```python
from build123d import *

# Parameters (mm, degrees)
BOSS_EXTRUDE1_DEPTH = 53.1
SKETCH3_W           = 0.955506131
SKETCH3_H           = 0.5
BOSS_EXTRUDE3_DEPTH = 5
BOSS_EXTRUDE4_DEPTH = 6
BOSS_EXTRUDE5_DEPTH = 5.84


with BuildPart() as part:
    # Sketch1 → Boss-Extrude1 (new body)
    with BuildSketch(Plane(origin=(0, 0, 0), x_dir=(0, 0, -1), z_dir=(1, 0, 0))):
        Polygon((0, 0), (12.5, 0), (12.5, 3.577441077), (3.577441077, 3.577441077), (3.577441077, 12.5), (0, 12.5), align=None)
    extrude(amount=BOSS_EXTRUDE1_DEPTH)

    # Sketch3 → Boss-Extrude3 (add)
    with BuildSketch(Plane.XZ):
        with Locations((1.917753066, -9.5)):
            Rectangle(SKETCH3_W, SKETCH3_H)
        with Locations((4.142246935, -9.5)):
            Rectangle(SKETCH3_W, SKETCH3_H)
        with Locations((48.957753066, -9.5)):
            Rectangle(SKETCH3_W, SKETCH3_H)
        with Locations((51.182246935, -9.5)):
            Rectangle(SKETCH3_W, SKETCH3_H)
    extrude(amount=BOSS_EXTRUDE3_DEPTH)

    # Sketch4 → Boss-Extrude4 (add)
    with BuildSketch(Plane.XY):
        Polygon((4.177995884, 4.261612802), (5.325991768, 6.25), (4.177995884, 8.238387198), (1.882004116, 8.238387198), (0.734008232, 6.25), (1.882004116, 4.261612802), align=None)
        Polygon((51.217995884, 4.261612802), (52.365991768, 6.25), (51.217995884, 8.238387198), (48.922004116, 8.238387198), (47.774008232, 6.25), (48.922004116, 4.261612802), align=None)
    extrude(amount=BOSS_EXTRUDE4_DEPTH)

    # Sketch6 → Boss-Extrude5 (add)
    with BuildSketch(Plane.XY):
        with BuildLine():
            Line((9.7116, 10.93), (43.3884, 10.93))
            ThreePointArc((43.3884, 10.93), (45.795005223, 9.807781555), (46.482272037, 7.242866885))
            Line((46.482272037, 7.242866885), (45.939749183, 4.166066885))
            ThreePointArc((45.939749183, 4.166066885), (44.8652587, 2.304994777), (42.845877146, 1.57))
            Line((42.845877146, 1.57), (10.254122854, 1.57))
            ThreePointArc((10.254122854, 1.57), (8.2347413, 2.304994777), (7.160250817, 4.166066885))
            Line((7.160250817, 4.166066885), (6.617727963, 7.242866885))
            ThreePointArc((6.617727963, 7.242866885), (7.304994777, 9.807781555), (9.7116, 10.93))
        make_face()
        with BuildLine():
            Line((9.7116, 10.43), (43.3884, 10.43))
            ThreePointArc((43.3884, 10.43), (45.411983001, 9.48638775), (45.98986816, 7.329690974))
            Line((45.98986816, 7.329690974), (45.447345306, 4.252890974))
            ThreePointArc((45.447345306, 4.252890974), (44.543864896, 2.688016999), (42.845877146, 2.07))
            Line((42.845877146, 2.07), (10.254122854, 2.07))
            ThreePointArc((10.254122854, 2.07), (8.556135104, 2.688016999), (7.652654694, 4.252890974))
            Line((7.652654694, 4.252890974), (7.11013184, 7.329690974))
            ThreePointArc((7.11013184, 7.329690974), (7.688016999, 9.48638775), (9.7116, 10.43))
        make_face(mode=Mode.SUBTRACT)
    extrude(amount=BOSS_EXTRUDE5_DEPTH)


solid = part.part
```
Geometry check sheet. Reference: the model listing, model coordinates, mm. A direction names the side the tool comes from. Round coordinates to 2 decimals unless told otherwise and drop trailing zeros. Order: outer loops, then holes, each group sorted by start corner. A loop starts at its lowest first (then second) coordinate and runs counter-clockwise, first axis right, second up. Notation, with made-up numbers: (77, -16.5) -> (130, -16.5) arc R12 ccw to (130, 6.5) -> close; hole circle Ø6 at (42, 28). An arc over 180 degrees is marked (long way). Return JSON: item names as keys, results as strings. Group by question number.
Q1. Section check A-A, the plane z = 2. Record the boundary of the cut face in (x, y), plus the area to 3 significant figures.
Q2. Section check D-D, the plane z = -7. Record the boundary of the cut face in (x, y).
Q3. Tool access check on faces 5 (the flat face through (0, 5, -3)), 6 (the flat face through (51.8, 7.23, 2.96)), 7 (the flat face through (4, -2, -9.25)), 8 (the flat face through (49, -2, -9.75)), 9 (the flat face through (7.385, 5.77, 2.879)). Record the directions out of +Z, -Z, +X, -X, +Y, -Y that give a thin tool (end or side, any length) a straight path to the whole face; none if there is none.
Q4. Section check B-B, the plane y = -3. Record the boundary of the cut face in (x, z).
Q5. Material ranges on probe 1 along Y at (x, z) = (32.5, 1.25); probe 2 along X at (y, z) = (5, 3.5); probe 3 along Y at (x, z) = (45.5, -3.25), recorded low to high. Write a range as from..to.
Q6. Section check C-C, the plane x = 21.5. Record the boundary of the cut face in (y, z).
Q7. Release check for a two-part mould opening along Y. For faces 1 (the flat face through (26, 8, -3.577)), 2 (the flat face through (26, 10.93, 3)), 3 (the flat face through (6.893, 5.683, 2.879)), 4 (the cylindrical face through (7.7, 9.5, 2.9)) record: released by +Y, released by -Y, zero draft, split by the parting line, or undercut.
Q8. Gauge pin test, flat ends, axial feed: pin 1 (6.5 mm diameter, centred on x = 28.5, z = 4.5, fed in from +Y); pin 2 (2.5 mm diameter, centred on x = 20, y = 7, fed in from -Z); pin 3 (0.7 mm diameter, centred on x = 50, z = 1.5, fed in from +Y); pin 4 (1 mm diameter, centred on y = 5, z = -8, fed in from +X). Record the tip position at first contact, or that the pin passes through.
Numbers:
{
 "1": {"outline": "(0.73, 6.25) -> (1.88, 4.26) -> (4.18, 4.26) -> (5.33, 6.25) -> (4.18, 8.24) -> (1.88, 8.24) -> close; (6.62, 7.24) -> (7.16, 4.17) arc R3.14 ccw to (10.25, 1.57) -> (42.85, 1.57) arc R3.14 ccw to (45.94, 4.17) -> (46.48, 7.24) arc R3.14 ccw to (43.39, 10.93) -> (9.71, 10.93) arc R3.14 ccw to start; (47.77, 6.25) -> (48.92, 4.26) -> (51.22, 4.26) -> (52.37, 6.25) -> (51.22, 8.24) -> (48.92, 8.24) -> close; hole (7.11, 7.33) -> (7.65, 4.25) arc R2.64 ccw to (10.25, 2.07) -> (42.85, 2.07) arc R2.64 ccw to (45.45, 4.25) -> (45.99, 7.33) arc R2.64 ccw to (43.39, 10.43) -> (9.71, 10.43) arc R2.64 ccw to start", "area": "72.7 mm^2"},
 "2": {"outline": "(0, 0) -> (53.1, 0) -> (53.1, 3.58) -> (0, 3.58) -> close"},
 "3": {"face 5": "+Z, -Z, -X, +Y, -Y", "face 6": "+Z, +X, +Y", "face 7": "+Z, +X, -X, -Y", "face 8": "-Z, +X, -X, -Y", "face 9": "+Z"},
 "4": {"outline": "(1.44, -9.75) -> (2.4, -9.75) -> (2.4, -9.25) -> (1.44, -9.25) -> close; (3.66, -9.75) -> (4.62, -9.75) -> (4.62, -9.25) -> (3.66, -9.25) -> close; (48.48, -9.75) -> (49.44, -9.75) -> (49.44, -9.25) -> (48.48, -9.25) -> close; (50.7, -9.75) -> (51.66, -9.75) -> (51.66, -9.25) -> (50.7, -9.25) -> close"},
 "5": {"probe 1": "1.57..2.07, 10.43..10.93", "probe 2": "1.46..4.6, 7.01..7.52, 45.58..46.09, 48.5..51.64", "probe 3": "0..12.5"},
 "6": {"outline": "(0, -12.5) -> (3.58, -12.5) -> (3.58, -3.58) -> (12.5, -3.58) -> (12.5, 0) -> (10.93, 0) -> (10.93, 5.84) -> (10.43, 5.84) -> (10.43, 0) -> (2.07, 0) -> (2.07, 5.84) -> (1.57, 5.84) -> (1.57, 0) -> (0, 0) -> close"},
 "7": {"face 1": "zero draft", "face 2": "released by +Y", "face 3": "released by -Y", "face 4": "undercut"},
 "8": {"pin 1": "y = 10.93", "pin 2": "z = -3.58", "pin 3": "y = 8.24", "pin 4": "through"}
}
